```python
from build123d import *

# Parameters (mm, degrees)
BOSS_EXTRUDE1_DEPTH = 1
SKETCH2_R           = 5
BOSS_EXTRUDE2_DEPTH = 1.4
SKETCH3_R           = 2.5
CUT_EXTRUDE1_DEPTH  = 8


with BuildPart() as part:
    # Sketch1 → Boss-Extrude1 (new body)
    with BuildSketch(Plane.XY):
        with BuildLine():
            ThreePointArc((-2.00408914, 4.838299183), (-6.471230468, 3.194539552), (-10, 0))
            ThreePointArc((-10, 0), (-9.238795325, -3.826834324), (-7.071067812, -7.071067812))
            ThreePointArc((-7.071067812, -7.071067812), (-2.316970366, -6.834731526), (2.00408914, -4.838299183))
            ThreePointArc((2.00408914, -4.838299183), (6.471230468, -3.194539552), (10, 0))
            ThreePointArc((10, 0), (9.238795325, 3.826834324), (7.071067812, 7.071067812))
            ThreePointArc((7.071067812, 7.071067812), (2.316970366, 6.834731526), (-2.00408914, 4.838299183))
        make_face()
    extrude(amount=BOSS_EXTRUDE1_DEPTH)

    # Sketch2 → Boss-Extrude2 (add)
    with BuildSketch(Plane.XY.offset(1)):
        Circle(SKETCH2_R)
    extrude(amount=BOSS_EXTRUDE2_DEPTH)

    # Sketch3 → Cut-Extrude1 (cut)
    with BuildSketch(Plane.XY.offset(2.4)):
        Circle(SKETCH3_R)
    extrude(amount=-CUT_EXTRUDE1_DEPTH, mode=Mode.SUBTRACT)


solid = part.part
```
Geometry check sheet. Reference: the model listing, model coordinates, mm. A direction names the side the tool comes from. Round coordinates to 2 decimals unless told otherwise and drop trailing zeros. Write each loop counter-clockwise with the first axis right and the second up, starting at its lowest first coordinate (ties: lowest second). Pieces come first, ordered by that corner, then holes. Notation, with made-up numbers: (53.5, 29.25) - (66.5, 29.25) arc R22 ccw to (66.5, 49.25) - close; hole circle Ø9 at (-23, 87). An arc over 180 degrees is marked (long way). Write each question's results on one line, items separated by ' | '.
(1) Set-up check for faces 5 (the face through (4.3, -3.1, 1)), 6 (the face through (2.38, 6.85, 0.49)): record each of +Z, -Z, +X, -X, +Y, -Y from which the full face is reachable in a straight line by a thin tool's end or side.
Computed:
face 5: +Z | face 6: +Z, -Z, +Y
(2) Draft check along Y on faces 1 (the face through (-1.08, -4.88, 1.69)), 2 (the face through (-0.54, -2.44, 1.22)), 3 (the face through (2, 2, 0)), 4 (the face through (9.26, 3.78, 0.49)). Enter one of: pulls with the +Y half, pulls with the -Y half, needs draft (parallel to the pull), parting line crosses it, or undercut.
Computed:
face 1: parting line crosses it | face 2: undercut | face 3: needs draft | face 4: pulls with the +Y half
(3) Thickness scan on probe 1 along Z at (x, y) = (-4.5, 2.5); probe 2 along Y at (x, z) = (0, 0.5); probe 3 along X at (y, z) = (-1, 1.95). Record the ranges inside material, lowest first. Write a range as from..to.
Computed:
probe 1: z = 0..1 | probe 2: y = -6.02..-2.5, 2.5..6.02 | probe 3: x = -4.9..-2.29, 2.29..4.9
(4) Depth check by flat-ended pin: pin 1 Ø1 at (x, z) = (-7.5, 0.5) entering from +Y; pin 2 Ø3 at (x, y) = (7.5, -3.5) entering from +Z. Enter the tip coordinate at first touch or a pass-through.
Computed:
pin 1: stops at y = 2.86 | pin 2: stops at z = 1
(5) Sectioned sample at B-B, the plane y = 1.25. Enter the section's corners in (x, z), plus the area to 3 significant figures.
Computed:
outline: (-8.93, 0) - (-2.17, 0) - (-2.17, 2.4) - (-4.84, 2.4) - (-4.84, 1) - (-8.93, 1) - close; (2.17, 0) - (9.92, 0) - (9.92, 1) - (4.84, 1) - (4.84, 2.4) - (2.17, 2.4) - close | area: 22.0 mm^2
(6) Sectioned sample at D-D, the plane y = 4.25. Enter the section's corners in (x, z).
Computed:
outline: (-4.26, 0) - (9.05, 0) - (9.05, 1) - (2.63, 1) - (2.63, 2.4) - (-2.63, 2.4) - (-2.63, 1) - (-4.26, 1) - close
(7) Sectioned sample at A-A, the plane z = 0.5. Enter the section's corners in (x, y).
Computed:
outline: (-10, 0) arc R10 ccw to (-7.07, -7.07) arc R12.5 ccw to (2, -4.84) arc R12.5 ccw to (10, 0) arc R10 ccw to (7.07, 7.07) arc R12.5 ccw to (-2, 4.84) arc R12.5 ccw to start; hole circle Ø5 at (0, 0)
(8) Sectioned sample at C-C, the plane x = 0. Enter the section's corners in (y, z), plus the area to 3 significant figures.
Computed:
outline: (-6.02, 0) - (-2.5, 0) - (-2.5, 2.4) - (-5, 2.4) - (-5, 1) - (-6.02, 1) - close; (2.5, 0) - (6.02, 0) - (6.02, 1) - (5, 1) - (5, 2.4) - (2.5, 2.4) - close | area: 14.0 mm^2
